Part model, mm, in its own coordinate system. A direction names the side the tool comes from. Give positions to 0.01 mm unless a question says otherwise; leave off trailing zeros. Write each loop counter-clockwise with the first axis right and the second up, starting at its lowest first coordinate (ties: lowest second). Pieces come first, ordered by that corner, then holes. Notation, with made-up numbers: (52, -27) - (90, -27) arc R15 ccw to (90, -16) - close; hole circle Ø10 at (-34.75, 65). An arc over 180 degrees is marked (long way). Answer in a Markdown table with one row per item. Add a question column.
1. Which spindle directions (+Z, -Z, +X, -X, +Y, -Y) get a long thin tool onto all of the face, cutting with end or side? Do faces 1 (the flat face through (0, 12, 17)), 2 (the flat face through (17, 12, 0)), 3 (the flat face through (-17, 12, 0)), 4 (the flat face through (0, 12, -17)). Say none if no direction does.
2. Pull direction Y, two halves, no side cores. Call faces 5 (the cylindrical face through (0.28, 159.298, 13.987)), 6 (the flat face through (-20, 94, 0)), 7 (the cylindrical face through (13.916, 134.094, 1.432)): released by +Y, released by -Y, zero draft, split by the parting line, or undercut.
3. Band-saw the part on B-B on y = 12. Write the cut outline in (x, z).
4. Probe line 1 along Y through (x, z) = (11, 0); line 2 along Z through (x, y) = (15.75, 145); line 3 along Y through (x, z) = (13.5, 4). List the from-to ranges inside material, lowest first.
5. Drop flat-ended pins along their axis: pin 1 Ø20 at (y, z) = (6.5, 2) entering from -X; pin 2 Ø20 at (x, y) = (-8, 13) entering from +Z; pin 3 Ø6 at (x, z) = (11.5, 9.5) entering from +Y. Give the stop position or say it passes through.
Autodesk Fusion 360 part; units mm, degrees
sketch "Sketch1" plane through (0, 0, 0) normal (0, 1, 0) x (1, 0, 0)
  line L0 (0, 17) -> (17, 17)
  line L1 (17, 17) -> (17, -17)
  line L2 (17, -17) -> (-17, -17)
  line L3 (-17, -17) -> (-17, 17)
  line L4 (-17, 17) -> (0, 17)
  dimension "d4" = 34
  dimension "d5" = 34
extrude "Extrude1" add sketch "Sketch1" along normal blind 25
sketch "Sketch2" plane through (0, 25, 0) normal (0, 1, 0) x (-1, 0, 0)
  line L0 (17, -17) -> (17, 17)
  line L1 (17, 17) -> (-17, 17)
  line L2 (-17, 17) -> (-17, -17)
  line L3 (-17, -17) -> (17, -17)
  line L4 (0, -20) -> (20, -20)
  line L5 (20, -20) -> (20, 20)
  line L6 (20, 20) -> (-20, 20)
  line L7 (-20, 20) -> (-20, -20)
  line L8 (-20, -20) -> (0, -20)
  dimension "d12" = 40
extrude "Extrude2" add sketch "Sketch2" along normal blind 140 contours L0 L1 L2 L3 | L4 L5 L6 L7 L8
sketch "Sketch3" plane through (0, 165, 0) normal (0, 1, 0) x (-1, 0, 0)
  line L0 (-20, -20) -> (20, -20)
  line L1 (20, -20) -> (20, 20)
  line L2 (20, 20) -> (-20, 20)
  line L3 (-20, 20) -> (-20, -20)
  line L4 (0, -17) -> (17, -17)
  line L5 (17, -17) -> (17, 17)
  line L6 (17, 17) -> (-17, 17)
  line L7 (-17, 17) -> (-17, -17)
  line L8 (-17, -17) -> (0, -17)
  dimension "d19" = 34
extrude "Extrude3" cut sketch "Sketch3" against normal blind 25 contours L4 L5 L6 L7 L8
extrude "Extrude4" add 1 faces at (5.6667, 140, -5.6667) along direction (0, 1, 0) blind 25
fillet "Fillet1" radius 20 2 edges at (0, 165, 20) (0, 165, -20)
hole "Hole1" at (20, 145, 0) direction (-1, 0, 0) diameter 22 depth 12 tip angle 118
Values:
| question | item | result |
|---|---|---|
| 1 | face 1 | +Z, +X, -X, -Y |
| 1 | face 2 | +Z, -Z, +X, -Y |
| 1 | face 3 | +Z, -Z, -X, -Y |
| 1 | face 4 | -Z, +X, -X, -Y |
| 2 | face 5 | released by +Y |
| 2 | face 6 | zero draft |
| 2 | face 7 | undercut |
| 3 | outline | (-17, -17) - (17, -17) - (17, 17) - (-17, 17) - close |
| 4 | line 1 | y = 0 to 134, 156 to 165 |
| 4 | line 2 | z = -20 to -11, 11 to 20 |
| 4 | line 3 | y = 0 to 134.75, 155.25 to 164.6 |
| 5 | pin 1 | stops at x = -17 |
| 5 | pin 2 | stops at z = 17 |
| 5 | pin 3 | stops at y = 163.92 |
